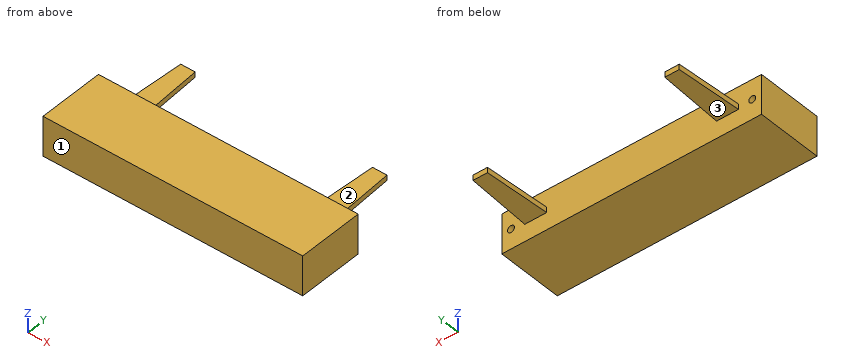
from build123d import *

# Parameters (mm, degrees)
SKETCH1_W                 = 60.198
SKETCH1_H                 = 9.1694
BOSS_EXTRUDE1_DEPTH       = 15.24
SKETCH2_W                 = 5.08
SKETCH2_H                 = 1.2192
BOSS_EXTRUDE2_DEPTH       = 15.24
CUT_EXTRUDE1_REACH        = 69.674
M2X0_4_TAPPED_HOLE1_D     = 1.6
M2X0_4_TAPPED_HOLE1_DEPTH = 2.567311505
M2X0_4_TAPPED_HOLE1_TIP   = 0.480688495


with BuildPart() as part:
    # Sketch1 → Boss-Extrude1 (new body)
    with BuildSketch(Plane(origin=(0, 0, 0), x_dir=(1, 0, 0), z_dir=(0, 1, 0))):
        with Locations((30.099, 4.5847)):
            Rectangle(SKETCH1_W, SKETCH1_H)
    extrude(amount=BOSS_EXTRUDE1_DEPTH)

    # Sketch2 → Boss-Extrude2 (add)
    with BuildSketch(Plane(origin=(0, 15.24, 0), x_dir=(1, 0, 0), z_dir=(0, 1, 0))):
        with Locations((7.874, 4.5847)):
            Rectangle(SKETCH2_W, SKETCH2_H)
        with Locations((52.324, 4.5847)):
            Rectangle(SKETCH2_W, SKETCH2_H)
    extrude(amount=BOSS_EXTRUDE2_DEPTH)

    # Sketch3 → Cut-Extrude1 (cut, up to next)
    with BuildSketch(Plane.XY.offset(-3.9751), mode=Mode.PRIVATE) as cut_extrude1_sk1:
        Polygon((5.334, 15.24), (6.1976, 30.48), (5.334, 30.48), align=None)
    cut_extrude1_tool1 = extrude(cut_extrude1_sk1.sketch, amount=-CUT_EXTRUDE1_REACH, mode=Mode.PRIVATE) & part.part
    # Sketch3 → Cut-Extrude1 (cut, up to next)
    with BuildSketch(Plane.XY.offset(-3.9751), mode=Mode.PRIVATE) as cut_extrude1_sk2:
        Polygon((10.414, 30.48), (9.5504, 30.48), (10.414, 15.24), align=None)
    cut_extrude1_tool2 = extrude(cut_extrude1_sk2.sketch, amount=-CUT_EXTRUDE1_REACH, mode=Mode.PRIVATE) & part.part
    cut_extrude1_1 = cut_extrude1_tool1.solids().sort_by_distance((5.621867, 25.4, -3.9751))[0]
    add(cut_extrude1_1, mode=Mode.SUBTRACT)
    cut_extrude1_2 = cut_extrude1_tool2.solids().sort_by_distance((10.126133, 25.4, -3.9751))[0]
    add(cut_extrude1_2, mode=Mode.SUBTRACT)
    cut_extrude1 = cut_extrude1_1 + cut_extrude1_2  # Cut-Extrude1 as one shape, for the pattern or mirror that repeats it

    # Mirror1: Cut-Extrude1 across plane
    add(cut_extrude1.mirror(Plane(origin=(30.099, 0, 0), x_dir=(0, 0, 1), z_dir=(1, 0, 0))), mode=Mode.SUBTRACT)

    # M2x0.4 Tapped Hole1
    with Locations(Plane(origin=(0, 15.24, 0), x_dir=(1, 0, 0), z_dir=(0, 1, 0))):
        with Locations((2.1336, 4.5847), (58.0644, 4.5847)):
            Hole(M2X0_4_TAPPED_HOLE1_D / 2, depth=M2X0_4_TAPPED_HOLE1_DEPTH)
            with Locations((0, 0, -(M2X0_4_TAPPED_HOLE1_DEPTH + M2X0_4_TAPPED_HOLE1_TIP / 2))):  # 118° drill point
                Cone(0, M2X0_4_TAPPED_HOLE1_D / 2, M2X0_4_TAPPED_HOLE1_TIP, mode=Mode.SUBTRACT)


solid = part.part
Input: part model. Units: mm. Frame: model coordinates. Face numbers are marked on the shaded views. A direction names the side the tool comes from. Give positions to 0.01 mm unless a question says otherwise; leave off trailing zeros. Loops run counter-clockwise (first coordinate to the right, second up) from the corner with the lowest first, then second, coordinate; pieces in that order, holes last. Notation, with made-up numbers: (43.5, 25) -> (95.5, 25) arc R17 ccw to (95.5, 48) -> close; hole circle Ø4 at (-10.5, 33.5). An arc over 180 degrees is marked (long way). Answer as a JSON object with one key per item and string values. Group by question number.
Item 1: Line query: probe 1 along Y at (x, z) = (9, -2.5). Output: solid intervals per line, ascending.
Item 2: Cut plane A-A, the plane y = 17.5. Return the cut outline in (x, z), and give its area (3 significant figures).
Item 3: Pin query (flat end, axial travel): P1, Ø4, axis at x = 8.5, y = 23.5, coming from the -Z side; P2, Ø1.5, axis at x = 6.5, y = 24.5, coming from the +Z side; P3, Ø1.4, axis at x = 2.13, z = -4.58, coming from the +Y side. Return the tip coordinate at first contact, or that it passes through.
Item 4: Cut plane C-C, the plane z = -7.25. Return the cut outline in (x, y).
Item 5: Cut plane B-B, the plane x = 7. Return the cut outline in (y, z), and give its area (3 significant figures).
Item 6: Reachability of the marked faces 1, 2 and 3 from +Z, -Z, +X, -X, +Y, -Y: full face, straight path, thin tool, end or side. Return the list, or none.
Item 7: Cut plane D-D, the plane x = 16.5. Return the cut outline in (y, z), and give its area (3 significant figures).
Checks:
{
 "1": {"probe 1": "y = 0 to 15.24"},
 "2": {"outline": "(5.46, -5.19) -> (10.29, -5.19) -> (10.29, -3.98) -> (5.46, -3.98) -> close; (49.91, -5.19) -> (54.74, -5.19) -> (54.74, -3.98) -> (49.91, -3.98) -> close", "area": "11.8 mm²"},
 "3": {"P1": "stops at z = -5.19", "P2": "stops at z = -3.98", "P3": "stops at y = 12.62"},
 "4": {"outline": "(0, 0) -> (60.2, 0) -> (60.2, 15.24) -> (0, 15.24) -> close"},
 "5": {"outline": "(0, -9.17) -> (15.24, -9.17) -> (15.24, -5.19) -> (30.48, -5.19) -> (30.48, -3.98) -> (15.24, -3.98) -> (15.24, 0) -> (0, 0) -> close", "area": "158 mm²"},
 "6": {"face 1": "+Z, -Z, +X, -X, -Y", "face 2": "+Z, +X, -X, +Y", "face 3": "-Z, +X, -X, +Y"},
 "7": {"outline": "(0, -9.17) -> (15.24, -9.17) -> (15.24, 0) -> (0, 0) -> close", "area": "140 mm²"}
}
